Here's how the part is built. I have some questions about the finished solid (model axes, mm). A direction names the side the tool comes from. Round coordinates to 2 decimals unless told otherwise and drop trailing zeros. Write each loop counter-clockwise with the first axis right and the second up, starting at its lowest first coordinate (ties: lowest second). Pieces come first, ordered by that corner, then holes. Notation, with made-up numbers: M 58,-13 L 96,-13 A25 ccw 96,23 Z; hole C 63.25,-23.75 d10. An arc over 180 degrees is marked long. Use one line per item in the form item = value. Start each with the question number.
Q1. I want a section at D-D on x = 3.5. List the corners of the cut face in (y, z) for me.
Q2. I want a section at B-B on y = 0.75. List the corners of the cut face in (x, z) for me, and give its area (3 significant figures).
Q3. I want a section at C-C on x = 2. List the corners of the cut face in (y, z) for me.
Q4. We'd pull the mould along X, two halves only. Please class faces 1 (the face through (-0.59, 1.34, 7.4)), 2 (the face through (2, 2, 15)), 3 (the face through (1.871, 3.736, 7.395)): +X half, -X half, draft (parallel to the pull), parting line (faces both ways), or undercut.
Q5. I'm going to push flat-ended pins straight in: pin 1 Ø4 at (x, z) = (-1, 3.5) entering from +Y; pin 2 Ø1.5 at (x, y) = (-1, 1) entering from +Z; pin 3 Ø2 at (x, z) = (4.5, 9.5) entering from -Y; pin 4 Ø2 at (x, z) = (4, 7) entering from +Y. Where does each tip first touch, or does it pass through?
Q6. I need wall thicknesses on line 1 along Y through (x, z) = (1.25, 7.5); line 2 along Y through (x, z) = (3, 3); line 3 along X through (y, z) = (-0.5, 14.75). Which ranges of each line are inside material? Lowest first, please. Write a range as from..to.
Q7. I want a section at A-A on x = -0.75. List the corners of the cut face in (y, z) for me, and give its area (3 significant figures).
Q8. For faces 4 (the face through (1.827, 1.734, 7.395)), 5 (the face through (2, 2, 0)), which set-ups out of +Z, -Z, +X, -X, +Y, -Y let a thin tool reach every point of the face, with its end or its side?
```python
from build123d import *

# Parameters (mm, degrees)
F1_DEPTH = 15
F2_R     = 0.5


with BuildPart() as f1:
    # F0 (on Top) → F1 (new body)
    with BuildSketch(Plane.XY):
        with BuildLine():
            ThreePointArc((0.314997359, 1.625), (1.8064242174, 1.7355083888), (3.2638192562, 1.4))
            Line((3.2638192562, 1.4), (3.2638192562, -1.4))
            ThreePointArc((3.2638192562, -1.4), (1.8064242174, -1.7355083888), (0.314997359, -1.625))
            ThreePointArc((0.314997359, -1.625), (-0.7212203567, -1.3356293712), (-1.7574380725, -1.625))
            Line((-1.7574380725, -1.625), (-1.7574380725, -2.9842268265))
            ThreePointArc((-1.7574380725, -2.9842268265), (1.8043736859, -3.739767503), (5.2638192562, -2.604170276))
            Line((5.2638192562, -2.604170276), (5.2638192562, 2.604170276))
            ThreePointArc((5.2638192562, 2.604170276), (1.8043736859, 3.739767503), (-1.7574380725, 2.9842268265))
            Line((-1.7574380725, 2.9842268265), (-1.7574380725, 1.625))
            ThreePointArc((-1.7574380725, 1.625), (-0.7212203567, 1.3356293712), (0.314997359, 1.625))
        make_face()
    extrude(amount=F1_DEPTH)

    # F2
    f2_edges = [f1.edges().sort_by_distance(p)[0] for p in [
        (0.314997, 1.625, 7.5),
        (0.314997, -1.625, 7.5),
        (-1.757438, -1.625, 7.5),
        (-1.757438, -2.984227, 7.5),
        (5.263819, -2.60417, 7.5),
        (5.263819, 2.60417, 7.5),
        (-1.757438, 2.984227, 7.5),
        (-1.757438, 1.625, 7.5),
    ]]
    fillet(f2_edges, radius=F2_R)


solid = f1.part
```
Reported:
q1.outline = M -3.44,0 L 3.44,0 L 3.44,15 L -3.44,15 Z
q2.outline = M 3.26,0 L 5.26,0 L 5.26,15 L 3.26,15 Z
q2.area = 30.0 mm^2
q3.outline = M -3.73,0 L -1.72,0 L -1.72,15 L -3.73,15 Z; M 1.72,0 L 3.73,0 L 3.73,15 L 1.72,15 Z
q4.face_1 = undercut
q4.face_2 = draft
q4.face_3 = parting line
q5.pin_1 = 3.74
q5.pin_2 = 15
q5.pin_3 = -3.44
q5.pin_4 = 3.57
q6.line_1 = -3.75..-1.75, 1.75..3.75
q6.line_2 = -3.57..-1.5, 1.5..3.57
q6.line_3 = 3.26..5.26
q7.outline = M -3.4,0 L -1.34,0 L -1.34,15 L -3.4,15 Z; M 1.34,0 L 3.4,0 L 3.4,15 L 1.34,15 Z
q7.area = 62.0 mm^2
q8.face_4 = +Z, -Z
q8.face_5 = -Z, +X, -X, +Y, -Y
